Could you check a few things on this model? Use its own coordinates, in mm. Give positions to 0.01 mm unless a question says otherwise; leave off trailing zeros. Write each loop counter-clockwise with the first axis right and the second up, starting at its lowest first coordinate (ties: lowest second). Pieces come first, ordered by that corner, then holes. Notation, with made-up numbers: (-16, 62) - (22, 62) arc R22 cw to (22, 71) - close; hole circle Ø3 at (-0.5, 56). An arc over 180 degrees is marked (long way). Answer as CSV lines item,"result". Start each with the question number.
Q1. Imagine slicing it at B-B on z = 1513. List the corners of the cut face in (x, y) for me (3 decimals), and give its area (3 significant figures).
Q2. If I drill on line 1 along Z through (x, y) = (-38.5, 48.5); line 2 along Z through (x, y) = (43.5, 39.5); line 3 along Z through (x, y) = (3.5, -43), over which ranges is the centre line in solid material (lowest first)?
Q3. Will these pins go through, and if not, where does the flat tip stop? pin 1 Ø11 at (x, z) = (62, 2386) entering from +Y; pin 2 Ø10 at (y, z) = (-15.5, 439) entering from +X; pin 3 Ø1 at (x, y) = (-69.5, -57.5) entering from -Z; pin 4 Ø6 at (x, y) = (-61, 95.5) entering from -Z.
Q4. Imagine slicing it at A-A on z = 2073.5. List the corners of the cut face in (x, y) for me (3 decimals), and give its area (3 significant figures).
```python
from build123d import *

# Parameters (mm, degrees)
F3_DEPTH        = 38.1
F4_DEPTH        = 76.2
F5_DEPTH        = 60.325
F8_DEPTH        = 57.15
F8_COPIES_COUNT = 4


# Not quite as in the source:
# - a pattern or mirror of a feature is missing from the dataset's text; its kind, count and spacing are read off the source's solid


with BuildPart() as f1:
    # F0 (on Front) → F1 (revolve)
    with BuildSketch(Plane.XZ):
        with BuildLine():
            Line((0, 1803.4), (0, 0))
            Line((0, 0), (139.7, 0))
            Line((139.7, 0), (139.7, 127))
            Line((139.7, 127), (127, 127))
            ThreePointArc((127, 127), (121.7511748434, 142.4625402968), (108.1740037456, 151.5345159877))
            Line((108.1740037456, 151.5345159877), (60.325, 164.3556179))
            Line((60.325, 164.3556179), (60.325, 1803.4))
            Line((60.325, 1803.4), (0, 1803.4))
        make_face()
    revolve(axis=Axis((0, 0, 901.7), (0, 0, -1)))

    # F2 (on face) → F3 (cut)
    with BuildSketch(Plane(origin=(0, 0, 0), x_dir=(1, 0, 0), z_dir=(0, 0, -1))):
        with BuildLine():
            ThreePointArc((43.7065244499, -62.4193857748), (67.5902254882, -35.1852443285), (76.2, 0))
            ThreePointArc((76.2, 0), (67.5902254882, 35.1852443285), (43.7065244499, 62.4193857748))
            ThreePointArc((43.7065244499, 62.4193857748), (0, 76.2), (-43.7065244499, 62.4193857748))
            ThreePointArc((-43.7065244499, 62.4193857748), (-76.2, 0), (-43.7065244499, -62.4193857748))
            ThreePointArc((-43.7065244499, -62.4193857748), (0, -76.2), (43.7065244499, -62.4193857748))
        make_face()
    extrude(amount=-F3_DEPTH, mode=Mode.SUBTRACT)

    # F2 (on face) → F4 (cut)
    with BuildSketch(Plane(origin=(0, 0, 0), x_dir=(1, 0, 0), z_dir=(0, 0, -1))):
        with BuildLine():
            ThreePointArc((-43.7065244499, -62.4193857748), (-76.2, 0), (-43.7065244499, 62.4193857748))
            Line((-43.7065244499, 62.4193857748), (-80.1286281582, 114.4355405872))
            ThreePointArc((-80.1286281582, 114.4355405872), (-139.7, 0), (-80.1286281582, -114.4355405872))
            Line((-80.1286281582, -114.4355405872), (-43.7065244499, -62.4193857748))
        make_face()
        with BuildLine():
            ThreePointArc((43.7065244499, 62.4193857748), (67.5902254882, 35.1852443285), (76.2, 0))
            ThreePointArc((76.2, 0), (67.5902254882, -35.1852443285), (43.7065244499, -62.4193857748))
            Line((43.7065244499, -62.4193857748), (80.1286281582, -114.4355405872))
            ThreePointArc((80.1286281582, -114.4355405872), (123.915413395, -64.5062812689), (139.7, 0))
            ThreePointArc((139.7, 0), (123.915413395, 64.5062812689), (80.1286281582, 114.4355405872))
            Line((80.1286281582, 114.4355405872), (43.7065244499, 62.4193857748))
        make_face()
    extrude(amount=-F4_DEPTH, mode=Mode.SUBTRACT)

    # F0 (on Front) → F5 (join, symmetric)
    with BuildSketch(Plane.XZ):
        Polygon((-60.325, 1803.4), (0, 1803.4), (60.325, 1803.4), (60.325, 2159), (49.2125, 2159), (0, 2159), (-60.325, 2159), align=None)
    extrude(amount=F5_DEPTH, both=True)

    # F0 (on Front) → F6 (revolve)
    with BuildSketch(Plane.XZ):
        Polygon((0, 2159), (49.2125, 2159), (49.2125, 2311.4), (88.9, 2311.4), (88.9, 2425.7), (53.975, 2425.7), (53.975, 2368.55), (0, 2368.55), align=None)
    revolve(axis=Axis((0, 0, 2263.775), (0, 0, -1)))

    # F7 (on face) → F8 (cut, through all)
    with BuildSketch(Plane.XY.offset(2425.7)):
        with BuildLine():
            ThreePointArc((53.975, 0), (53.0995163948, -9.6820443933), (50.5014665629, -19.05))
            Line((50.5014665629, -19.05), (86.834944003, -19.05))
            ThreePointArc((86.834944003, -19.05), (88.3822281962, -9.5808005442), (88.9, 0))
            ThreePointArc((88.9, 0), (88.3822281962, 9.5808005442), (86.834944003, 19.05))
            Line((86.834944003, 19.05), (50.5014665629, 19.05))
            ThreePointArc((50.5014665629, 19.05), (53.0995163948, 9.6820443933), (53.975, 0))
        make_face()
    f8 = extrude(amount=-F8_DEPTH, mode=Mode.SUBTRACT)

    # F8_copies: F8 ×4 about axis
    f8_copies_axis = Axis((0, 0, 0), (0, 0, 1))
    for i in range(1, F8_COPIES_COUNT):
        add(f8.rotate(f8_copies_axis, i * 360 / F8_COPIES_COUNT), mode=Mode.SUBTRACT)


solid = f1.part
```
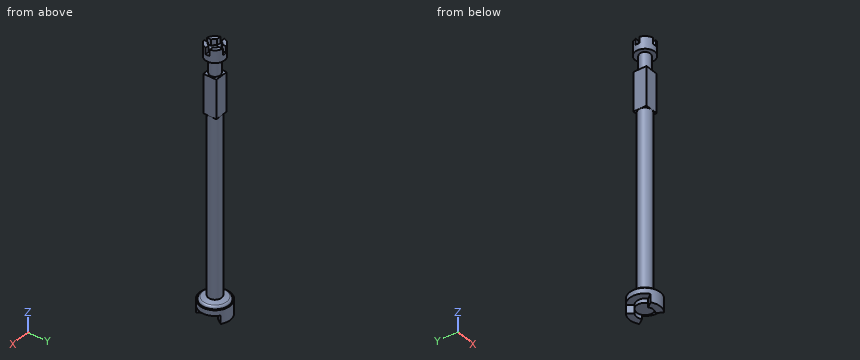
Conclusion:
1,outline,"circle Ø120.65 at (0, 0)"
1,area,"11,400 mm^2"
2,line 1,"38.1 to 163.93, 1803.4 to 2159, 2311.4 to 2425.7"
2,line 2,"38.1 to 2159, 2311.4 to 2425.7"
2,line 3,"38.1 to 2368.55"
3,pin 1,"y = 68.64"
3,pin 2,"x = 59.4"
3,pin 3,"z = 76.2"
3,pin 4,"z = 0"
4,outline,"(-60.325, -60.325) - (60.325, -60.325) - (60.325, 60.325) - (-60.325, 60.325) - close"
4,area,"14,600 mm^2"
